from build123d import *

# Parameters (mm, degrees)
F0_W     = 100
F0_H     = 150
F1_DEPTH = 14.6
F2_W     = 8
F2_H     = 150
F3_DEPTH = 1
F4_R     = 1.7
F5_DEPTH = 25


with BuildPart() as f1:
    # F0 (on Top) → F1 (new body)
    with BuildSketch(Plane.XY):
        with Locations((50, -75)):
            Rectangle(F0_W, F0_H)
    extrude(amount=F1_DEPTH)

    # F2 (on face) → F3 (cut)
    with BuildSketch(Plane.XY.offset(14.6)):
        with Locations((9, -75)):
            Rectangle(F2_W, F2_H)
        with Locations((19, -75)):
            Rectangle(F2_W, F2_H)
        with Locations((29, -75)):
            Rectangle(F2_W, F2_H)
        with Locations((39, -75)):
            Rectangle(F2_W, F2_H)
        with Locations((49, -75)):
            Rectangle(F2_W, F2_H)
        with Locations((59, -75)):
            Rectangle(F2_W, F2_H)
        with Locations((69, -75)):
            Rectangle(F2_W, F2_H)
        with Locations((79, -75)):
            Rectangle(F2_W, F2_H)
        with Locations((89, -75)):
            Rectangle(F2_W, F2_H)
    extrude(amount=-F3_DEPTH, mode=Mode.SUBTRACT)

    # F4 (on face) → F5 (cut)
    with BuildSketch(Plane.XY.offset(14.6)):
        with Locations((2.5, -2.5)):
            Circle(F4_R)
        with Locations((2.5, -147.5)):
            Circle(F4_R)
        with Locations((97.5, -147.5)):
            Circle(F4_R)
        with Locations((97.5, -2.5)):
            Circle(F4_R)
    extrude(amount=-F5_DEPTH, mode=Mode.SUBTRACT)


solid = f1.part
CAD build for the part. Positions are in the model's coordinates, mm. A direction names the side the tool comes from. Give positions to 0.01 mm unless a question says otherwise; leave off trailing zeros. Write each loop counter-clockwise with the first axis right and the second up, starting at its lowest first coordinate (ties: lowest second). Pieces come first, ordered by that corner, then holes. Notation, with made-up numbers: (66, 63.25) -> (124, 63.25) arc R18 ccw to (124, 69.25) -> close; hole circle Ø7 at (14, 11.5). An arc over 180 degrees is marked (long way). Return JSON: item names as keys, results as strings.
Item 1: Band-saw the part on B-B (y = -147.5). Give the number of separate pieces and of enclosed holes in the cut face, then the cut area to 3 significant figures.
Answer below:
{"separate pieces": "3", "enclosed holes": "0", "area": "1,290 mm2"}
Item 2: Band-saw the part on A-A (x = 2.5). List the corners of the cut face in (y, z), then the cut area to 3 significant figures.
Answer below:
{"outline": "(-150, 0) -> (-149.2, 0) -> (-149.2, 14.6) -> (-150, 14.6) -> close; (-145.8, 0) -> (-4.2, 0) -> (-4.2, 14.6) -> (-145.8, 14.6) -> close; (-0.8, 0) -> (0, 0) -> (0, 14.6) -> (-0.8, 14.6) -> close", "area": "2,090 mm2"}
Item 3: Drop a flat-ended pin along its axis: pin 1 (2.5 mm diameter, centred on x = 59.5, y = -55.5, fed in from +Z). Give the stop position or say it passes through.
Answer below:
{"pin 1": "stops at z = 13.6"}
Item 4: Tool access for faces 5 (the flat face through (96, -74, 14.6)), 6 (the flat face through (59, -74, 13.6)): list every direction of +Z, -Z, +X, -X, +Y, -Y with a clear straight run to the whole face (end or side of a thin tool).
Answer below:
{"face 5": "+Z, +X, -X, +Y, -Y", "face 6": "+Z, +Y, -Y"}
Item 5: Two-plate mould, pull along Y, no slides. Class faces 1 (the flat face through (49, 0, 7)), 2 (the flat face through (49, -150, 7)), 3 (the cylindrical face through (4.12, -1.99, 7.4)), 4 (the flat face through (29, -74, 13.6)): +Y half, -Y half, draft (parallel to the pull), parting line (faces both ways), or undercut.
Answer below:
{"face 1": "+Y half", "face 2": "-Y half", "face 3": "undercut", "face 4": "draft"}
Item 6: Band-saw the part on C-C (x = 67.5). List the corners of the cut face in (y, z), then the cut area to 3 significant figures.
Answer below:
{"outline": "(-150, 0) -> (0, 0) -> (0, 13.6) -> (-150, 13.6) -> close", "area": "2,040 mm2"}
Item 7: Drill centre lines: probe 1 along X at (y, z) = (-147.5, 10); probe 2 along Y at (x, z) = (97.5, 6); probe 3 along Z at (x, y) = (37, -80). Where is each one in solid material? Low to high.
Answer below:
{"probe 1": "x = 0 to 0.8, 4.2 to 95.8, 99.2 to 100", "probe 2": "y = -150 to -149.2, -145.8 to -4.2, -0.8 to 0", "probe 3": "z = 0 to 13.6"}
